Autodesk Inventor part; units mm, degrees
ref_plane "YZ Plane" through (0, 0, 0) normal (1, 0, 0) x (0, 1, 0)
ref_plane "XZ Plane" through (0, 0, 0) normal (0, 1, 0) x (-1, 0, 0)
ref_plane "XY Plane" through (0, 0, 0) normal (0, 0, 1) x (1, 0, 0)
sketch "Sketch1" plane through (0, 0, 0) normal (0, 0, 1) x (1, 0, 0)
  arc A0 (37.4971, -0.4687) -> (-37.4971, -0.4688) centre (0, 0) ccw
  line L0 (0, 0) -> (0, -200) construction
  arc A1 (-35, -200) -> (35, -200) centre (0, -200) ccw
  circle A2 centre (0, -200) radius 4.75
  circle A3 centre (0, 0) radius 4.75
  line L1 (0, -200) -> (18.25, -200) construction
  circle A4 centre (18.25, -200) radius 2.5
  circle A5 centre (0, -200) radius 21 construction
  line L2 (0, -235) -> (0, -230) construction
  circle A6 centre (0, -230) radius 1.5
  line L3 (37.4971, -0.4687) -> (34.9973, -200.4375)
  line L4 (-37.4971, -0.4688) -> (-34.9973, -200.4375)
  line L5 (36.2472, -100.4531) -> (31.2476, -100.3906) construction
  line L6 (30.4976, -160.3859) -> (31.9976, -40.3953) construction
  circle A7 centre (31.9976, -40.3953) radius 1.5
  circle A8 centre (31.2476, -100.3906) radius 1.5
  circle A9 centre (30.4976, -160.3859) radius 1.5
  line L7 (37.5, 0) -> (32.5, 0) construction
  line L8 (0, 37.5) -> (0, 32.5) construction
  circle A10 centre (0, 32.5) radius 1.5
  circle A11 centre (32.5, 0) radius 1.5
  line L9 (35, -200) -> (30, -200) construction
  circle A12 centre (30, -200) radius 1.5
  circle A13 centre (-31.9976, -40.3953) radius 1.5
  circle A14 centre (-31.2476, -100.3906) radius 1.5
  circle A15 centre (-30.4976, -160.3859) radius 1.5
  circle A16 centre (-32.5, 0) radius 1.5
  line L10 (-35, -200) -> (-30, -200) construction
  circle A17 centre (-30, -200) radius 1.5
  line L11 (0, 0) -> (16, 0) construction
  circle A18 centre (16, 0) radius 2.5
  line L12 (0, -200) -> (-18.25, -200) construction
  circle A19 centre (-18.25, -200) radius 2.5
  line L13 (0, 0) -> (-16, 0) construction
  circle A20 centre (-16, 0) radius 2.5
  line L14 (0, -200) -> (0, -60.58) construction
  line L15 (0, -200) -> (47.7906, -152.2094) construction
  line L16 (0, -200) -> (0, -182) construction
  circle A21 centre (-8, -178.3533) radius 1.1
  circle A22 centre (-4.1372, -169.6741) radius 1.1
  dimension "D_Junta2" = 75
  dimension "L_Elo" = 200
  dimension "D_Junta3" = 70
  dimension "Veio" = 9.5
  dimension "d4" = 9.5
  dimension "d5" = 18.25
  dimension "d6" = 5
  dimension "D_P" = 42
  dimension "LF" = 5
  dimension "D_Sup" = 3
  dimension "d10" = 5
  dimension "d12" = 120
  dimension "d13" = 3
  dimension "d14" = 3
  dimension "d15" = 3
  dimension "d16" = 5
  dimension "d17" = 5
  dimension "d18" = 3
  dimension "d19" = 3
  dimension "d20" = 5
  dimension "d21" = 3
  dimension "d22" = 16
  dimension "d23" = 5
  dimension "d26" = 139.42
  dimension "d33" = 135
  dimension "d34" = 18
  dimension "d35" = 2.2
  dimension "d36" = 2.2
  dimension "d37" = 9.5
  dimension "d41" = 8
  dimension "d42" = 4.1372
  dimension "d43" = 21.6467
extrude "Extrusion1" add sketch "Sketch1" along normal blind 4 contours L3 A1 L4 A0 | A21 | A22
sketch "Sketch2" plane through (0, 0, 4) normal (0, 0, 1) x (1, 0, 0)
  line L0 (0, 0) -> (0, 36)
  line L1 (-0.005, 35.995) -> (0.005, 35.995)
  line L2 (0.005, 35.995) -> (0.005, 36.005)
  line L3 (0.005, 36.005) -> (-0.005, 36.005)
  line L4 (-0.005, 36.005) -> (-0.005, 35.995)
  line L5 (-0.005, 35.995) -> (0.005, 36.005) construction
  line L6 (0.005, 35.995) -> (-0.005, 36.005) construction
  dimension "d28" = 36
  dimension "d29" = 0.01
  dimension "d30" = 0.01
extrude "Extrusion2" add sketch "Sketch2" along normal blind 0.01
extrude "Extrusion3" cut sketch "Sketch1" along normal up to surface (4 mm away) contours A21 | A22
equation "\"d4\" = Veio"
equation "\"d10\" = LF"
equation "\"d13\" = D_Sup"
equation "\"d14\" = D_Sup"
equation "\"d15\" = D_Sup"
equation "\"d16\" = LF"
equation "\"d17\" = LF"
equation "\"d18\" = D_Sup"
equation "\"d19\" = D_Sup"
equation "\"d20\" = LF"
equation "\"d21\" = D_Sup"
properties part number "4ELO"
Part model, mm, in its own coordinate system. Round coordinates to 2 decimals unless told otherwise and drop trailing zeros. Order: outer loops, then holes, each group sorted by start corner. A loop starts at its lowest first (then second) coordinate and runs counter-clockwise, first axis right, second up. Notation, with made-up numbers: M 1,-16 L 24,-16 A16 cw 24,13 Z; hole C 26,46 d11. An arc over 180 degrees is marked long. Put each result on its own line as item: value. Start each with the question number.
1. Slice it at C-C on y = -216.5. List the corners of the cut face in (x, z).
2. Drop flat-ended pins along their axis: pin 1 (1 mm diameter, centred on y = -32, z = 2.5, fed in from -X); pin 2 (1 mm diameter, centred on y = -19, z = 1, fed in from +X); pin 3 (6 mm diameter, centred on x = -16, y = 0, fed in from +Z). Give the stop position or say it passes through.
3. Slice it at B-B on y = -81.5. List the corners of the cut face in (x, z).
4. Two-plate mould, pull along X, no slides. Class faces 1 (the face through (17.92, -202.48, 1.97)), 2 (the face through (-0.83, 37.49, 1.97)), 3 (the face through (-1, -97, 4)): +X half, -X half, draft (parallel to the pull), parting line (faces both ways), or undercut.
5. Drill centre lines: probe 1 along Y at (x, z) = (3.5, 3.25); probe 2 along Y at (x, z) = (-32.5, 1.1); probe 3 along Y at (x, z) = (-16.5, 0.7). Where is each one in solid material? Low to high. Write a range as [from, to].
6. Slice it at A-A on z = 2.3. State how many separate pieces and enclosed holes the cut face has, then the cut area to 3 significant figures.
Findings:
1. outline: M -30.87,0 L 30.87,0 L 30.87,4 L -30.87,4 Z
2. pin 1: x = -37.11
2. pin 2: x = 37.27
2. pin 3: z = 4
3. outline: M -36.48,0 L 36.48,0 L 36.48,4 L -36.48,4 Z
4. face 1: undercut
4. face 2: parting line
4. face 3: draft
5. probe 1: [-234.82, -203.21], [-196.79, -3.21], [3.21, 37.34]
5. probe 2: [-212.99, -101.22], [-99.57, -41.81], [-38.98, -1.5], [1.5, 18.71]
5. probe 3: [-230.87, -201.79], [-198.21, -2.45], [2.45, 33.67]
6. separate pieces: 1
6. enclosed holes: 20
6. area: 18,300 mm2
